```python
from build123d import *

# Parameters (mm, degrees)
CUT_EXTRUDE_1_DEPTH = 2
FILLET_1_R          = 0.3
CHAMFER_1_SIZE      = 1


with BuildPart() as part:
    # Эскиз1 → Повернуть1 (revolve)
    with BuildSketch(Plane.XY):
        Polygon((0, 0), (0, 4.9), (0.5, 4.9), (3, 2.5), (12, 2.5), (12, 0), align=None)
    revolve(axis=Axis((12, 0, 0), (-1, 0, 0)))

    # Эскиз2 → Вырез-Вытянуть1 (cut)
    with BuildSketch(Plane.ZY):
        Polygon((0.866025404, 1.5), (-0.866025404, 1.5), (-1.732050808, 0), (-0.866025404, -1.5), (0.866025404, -1.5), (1.732050808, 0), align=None)
    extrude(amount=-CUT_EXTRUDE_1_DEPTH, mode=Mode.SUBTRACT)

    # Скругление1
    fillet_1_edges = [part.edges().sort_by_distance(p)[0] for p in [
        (0, -4.9, 0),
    ]]
    fillet(fillet_1_edges, radius=FILLET_1_R)

    # Фаска1
    chamfer_1_edges = [part.edges().sort_by_distance(p)[0] for p in [
        (12, -2.5, 0),
    ]]
    chamfer(chamfer_1_edges, length=CHAMFER_1_SIZE)


solid = part.part
```
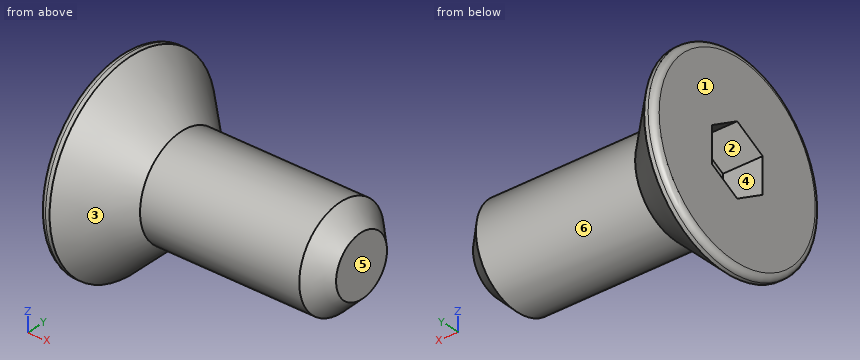
Geometry: final body of the model. Coordinates: model frame, mm. Face numbers are marked on the shaded views. A direction names the side the tool comes from. Round coordinates to 2 decimals unless told otherwise and drop trailing zeros. Write each loop counter-clockwise with the first axis right and the second up, starting at its lowest first coordinate (ties: lowest second). Pieces come first, ordered by that corner, then holes. Notation, with made-up numbers: (-24, -24) -> (16, -24) arc R27 cw to (16, -4) -> close; hole circle Ø11 at (-1, 22). An arc over 180 degrees is marked (long way). Use CSV: the item, a comma, the result in double quotes. Start each with the question number.
Q1. First-contact query: pin 1 Ø4 at (x, y) = (2.5, 3) entering from -Z; pin 2 Ø2 at (x, y) = (11, -1.5) entering from +Z; pin 3 Ø3 at (x, z) = (6, 1) entering from -Y. Flat tips, straight axial feed; report the tip coordinate or a pass-through.
Q2. Section B-B (x = 1). Return loops of the section in (y, z).
Q3. Reachability of the marked faces 4, 5 and 6 from +Z, -Z, +X, -X, +Y, -Y: full face, straight path, thin tool, end or side. Return the list, or none.
Q4. Pull-direction query (Y, two-part tool) for the marked faces 1, 2 and 3; classes: pulls with the +Y half, pulls with the -Y half, needs draft (parallel to the pull), parting line crosses it, or undercut.
Q5. Line query: L1, parallel to X at y = 0.5, z = -0.25; L2, parallel to Y at x = 4, z = -2; L3, parallel to X at y = 3.25, z = -3. Output: solid intervals per line, ascending.
Q6. Section C-C (x = 4.5). Return loops of the section in (y, z).
Q7. Section A-A (z = 0). Return loops of the section in (x, y), plus the area to 3 significant figures.
Result sheet:
1,pin 1,"z = -4.2"
1,pin 2,"z = 2.45"
1,pin 3,"y = -2.5"
2,outline,"circle Ø8.84 at (0, 0); hole (-1.5, -0.87) -> (0, -1.73) -> (1.5, -0.87) -> (1.5, 0.87) -> (0, 1.73) -> (-1.5, 0.87) -> close"
3,face 4,"-X"
3,face 5,"+Z, -Z, +X, +Y, -Y"
3,face 6,"+X"
4,face 1,"needs draft"
4,face 2,"undercut"
4,face 3,"parting line crosses it"
5,L1,"2 to 12"
5,L2,"-1.5 to 1.5"
5,L3,"0 to 1"
6,outline,"circle Ø5 at (0, 0)"
7,outline,"(0, -4.6) arc R0.3 ccw to (0.3, -4.9) -> (0.5, -4.9) -> (3, -2.5) -> (11, -2.5) -> (12, -1.5) -> (12, 1.5) -> (11, 2.5) -> (3, 2.5) -> (0.5, 4.9) -> (0.3, 4.9) arc R0.3 ccw to (0, 4.6) -> (0, 1.5) -> (2, 1.5) -> (2, -1.5) -> (0, -1.5) -> close"
7,area,"61.4 mm²"
